Work out the finished part from the listing and answer in its coordinate system (mm). Coordinates: 2 decimals unless noted, no trailing zeros. Order: outer loops, then holes, each group sorted by start corner. A loop starts at its lowest first (then second) coordinate and runs counter-clockwise, first axis right, second up. Notation, with made-up numbers: (38, -29.75) - (57, -29.75) arc R22 ccw to (57, -4.75) - close; hole circle Ø8 at (-8.75, 31). An arc over 180 degrees is marked (long way). Answer as a JSON object with one key per item and string values. Group by question number.
1) Section D-D (x = 7.25) is taken. Give the vertices of the cut face in (y, z).
2) Section C-C (y = -1.65) is taken. Give the vertices of the cut face in (x, z).
3) Section A-A (x = 0) is taken. Give the vertices of the cut face in (y, z), plus the area to 3 significant figures.
4) The mould has two halves that part along Z. Classify faces 1 (the face through (-10, -1, 1)), 2 (the face through (0, -1, -42)), 3 (the face through (0, -1, -50)), 4 (the face through (0, -1, 38)): released by +Z, released by -Z, zero draft, split by the parting line, or undercut.
5) Find the intervals of material crossed by line 1 along Z through (x, y) = (0, -1.7); line 2 along Z through (x, y) = (-1, -2.45); line 3 along X through (y, z) = (-2.25, -39.5), in increasing order.
6) Section B-B (z = 22) is taken. Give the vertices of the cut face in (x, y).
7) Each of these flat-tipped pins is pushed along its axis until it touches: P1, Ø1.5, axis at x = -5.5, y = -1, coming from the +Z side; P2, Ø2.5, axis at x = 0, z = -40, coming from the +Y side; P3, Ø1, axis at x = 6.5, y = -2, coming from the -Z side. Where does it stop, or does it pass through?
from build123d import *

# Parameters (mm, degrees)
F0_R     = 2
F1_DEPTH = 3


with BuildPart() as f1:
    # F0 (on Front) → F1 (new body)
    with BuildSketch(Plane.XZ):
        with BuildLine():
            ThreePointArc((-10, -40), (0, -50), (10, -40))
            Line((10, -40), (10, 40))
            ThreePointArc((10, 40), (0, 50), (-10, 40))
            Line((-10, 40), (-10, -40))
        make_face()
        with Locations((0, -40)):
            Circle(F0_R, mode=Mode.SUBTRACT)
        with Locations((0, 22)):
            Circle(F0_R, mode=Mode.SUBTRACT)
        with Locations((0, 40)):
            Circle(F0_R, mode=Mode.SUBTRACT)
    extrude(amount=F1_DEPTH)


solid = f1.part
Report:
{
 "1": {"outline": "(-3, -46.89) - (0, -46.89) - (0, 46.89) - (-3, 46.89) - close"},
 "2": {"outline": "(-10, -40) arc R10 ccw to (10, -40) - (10, 40) arc R10 ccw to (-10, 40) - close; hole circle Ø4 at (0, -40); hole circle Ø4 at (0, 22); hole circle Ø4 at (0, 40)"},
 "3": {"outline": "(-3, -50) - (0, -50) - (0, -42) - (-3, -42) - close; (-3, -38) - (0, -38) - (0, 20) - (-3, 20) - close; (-3, 24) - (0, 24) - (0, 38) - (-3, 38) - close; (-3, 42) - (0, 42) - (0, 50) - (-3, 50) - close", "area": "264 mm²"},
 "4": {"face 1": "zero draft", "face 2": "undercut", "face 3": "released by -Z", "face 4": "undercut"},
 "5": {"line 1": "z = -50 to -42, -38 to 20, 24 to 38, 42 to 50", "line 2": "z = -49.95 to -41.73, -38.27 to 20.27, 23.73 to 38.27, 41.73 to 49.95", "line 3": "x = -10 to -1.94, 1.94 to 10"},
 "6": {"outline": "(-10, -3) - (-2, -3) - (-2, 0) - (-10, 0) - close; (2, -3) - (10, -3) - (10, 0) - (2, 0) - close"},
 "7": {"P1": "stops at z = 48.8", "P2": "passes through", "P3": "stops at z = -48"}
}
